Here's how the part is built. I have some questions about the finished solid (model axes, mm). Face numbers are marked on the shaded views. A direction names the side the tool comes from. Round coordinates to 2 decimals unless told otherwise and drop trailing zeros. Order: outer loops, then holes, each group sorted by start corner. A loop starts at its lowest first (then second) coordinate and runs counter-clockwise, first axis right, second up. Notation, with made-up numbers: (-22, 1) - (-2, 1) arc R17 cw to (-2, 12) - close; hole circle Ø2 at (56, 82.25). An arc over 180 degrees is marked (long way). One line per item, written item: value.
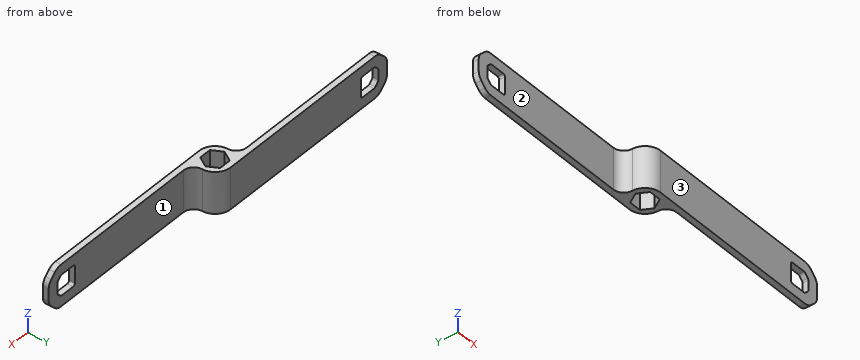
from build123d import *

# Parameters (mm, degrees)
SKETCH2_R           = 7.5
BOSS_EXTRUDE1_DEPTH = 20
SKETCH3_W           = 20
SKETCH3_H           = 2.7375
BOSS_EXTRUDE2_DEPTH = 90
FILLET1_R           = 5
CHAMFER1_SIZE       = 5
FILLET2_R           = 5
CUT_EXTRUDE1_DEPTH  = 45
FILLET3_R           = 1
SKETCH5_W           = 20
SKETCH5_H           = 2.7375
BOSS_EXTRUDE3_DEPTH = 90
CHAMFER2_SIZE       = 5
FILLET4_R           = 5
FILLET5_R           = 5
CUT_EXTRUDE2_DEPTH  = 90
FILLET6_R           = 1


with BuildPart() as part:
    # Sketch2 → Boss-Extrude1 (new body)
    with BuildSketch(Plane.XY):
        Circle(SKETCH2_R)
        Polygon((5.499261314, 0), (2.749630657, 4.7625), (-2.749630657, 4.7625), (-5.499261314, 0), (-2.749630657, -4.7625), (2.749630657, -4.7625), align=None, mode=Mode.SUBTRACT)
    extrude(amount=BOSS_EXTRUDE1_DEPTH)

    # Sketch3 → Boss-Extrude2 (add)
    with BuildSketch(Plane.ZY):
        with Locations((10, 6.13125)):
            Rectangle(SKETCH3_W, SKETCH3_H)
    extrude(amount=BOSS_EXTRUDE2_DEPTH)

    # Fillet1
    fillet1_edges = [part.edges().sort_by_distance(p)[0] for p in [
        (-5.793841019, 4.7625, 10),
    ]]
    fillet(fillet1_edges, radius=FILLET1_R)

    # Chamfer1
    chamfer1_edges = [part.edges().sort_by_distance(p)[0] for p in [
        (-90, 6.13125, 0),
        (-90, 6.13125, 20),
    ]]
    chamfer(chamfer1_edges, length=CHAMFER1_SIZE)

    # Fillet2
    fillet2_edges = [part.edges().sort_by_distance(p)[0] for p in [
        (-90, 6.13125, 15),
        (-90, 6.13125, 5),
        (-85, 6.13125, 0),
        (-85, 6.13125, 20),
    ]]
    fillet(fillet2_edges, radius=FILLET2_R)

    # Sketch4 → Cut-Extrude1 (cut)
    with BuildSketch(Plane(origin=(0, 7.5, 0), x_dir=(1, 0, 0), z_dir=(0, 1, 0))):
        Polygon((-74.928932188, -15), (-74.928932188, -5), (-82.928932188, -5), (-85, -7.071067812), (-85, -12.928932188), (-82.928932188, -15), align=None)
    extrude(amount=-CUT_EXTRUDE1_DEPTH, mode=Mode.SUBTRACT)

    # Fillet3
    fillet3_edges = [part.edges().sort_by_distance(p)[0] for p in [
        (-74.928932188, 6.13125, 15),
        (-82.928932188, 6.13125, 15),
        (-85, 6.13125, 12.928932188),
        (-85, 6.13125, 7.071067812),
        (-82.928932188, 6.13125, 5),
        (-74.928932188, 6.13125, 5),
    ]]
    fillet(fillet3_edges, radius=FILLET3_R)

    # Sketch5 → Boss-Extrude3 (add)
    with BuildSketch(Plane.ZY):
        with Locations((10, -6.13125)):
            Rectangle(SKETCH5_W, SKETCH5_H)
    extrude(amount=-BOSS_EXTRUDE3_DEPTH)

    # Chamfer2
    chamfer2_edges = [part.edges().sort_by_distance(p)[0] for p in [
        (90, -6.13125, 20),
        (90, -6.13125, 0),
    ]]
    chamfer(chamfer2_edges, length=CHAMFER2_SIZE)

    # Fillet4
    fillet4_edges = [part.edges().sort_by_distance(p)[0] for p in [
        (85, -6.13125, 20),
        (90, -6.13125, 5),
        (90, -6.13125, 15),
        (85, -6.13125, 0),
    ]]
    fillet(fillet4_edges, radius=FILLET4_R)

    # Fillet5
    fillet5_edges = [part.edges().sort_by_distance(p)[0] for p in [
        (5.793841019, -4.7625, 10),
    ]]
    fillet(fillet5_edges, radius=FILLET5_R)

    # Sketch7 → Cut-Extrude2 (cut)
    with BuildSketch(Plane.XZ.offset(7.5)):
        Polygon((74.928932188, 5), (74.928932188, 15), (82.928932188, 15), (85, 12.928932188), (85, 7.071067812), (82.928932188, 5), align=None)
    extrude(amount=-CUT_EXTRUDE2_DEPTH, mode=Mode.SUBTRACT)

    # Fillet6
    fillet6_edges = [part.edges().sort_by_distance(p)[0] for p in [
        (82.928932188, -6.13125, 5),
        (74.928932188, -6.13125, 5),
        (74.928932188, -6.13125, 15),
        (82.928932188, -6.13125, 15),
        (85, -6.13125, 12.928932188),
        (85, -6.13125, 7.071067812),
    ]]
    fillet(fillet6_edges, radius=FILLET6_R)


solid = part.part
Q1. If I drill on line 1 along Y through (x, z) = (-26.5, 10.5); line 2 along Y through (x, z) = (45.5, 3); line 3 along X through (y, z) = (2, 9.25), over which ranges is the centre line in solid material (lowest first)?
Results list:
line 1: 4.76 to 7.5
line 2: -7.5 to -4.76
line 3: -8.03 to -4.34, 4.34 to 7.23
Q2. If we section it at A-A, the plane x = -54: Please give me the cut outline in (y, z).
Results list:
outline: (4.76, 0) - (7.5, 0) - (7.5, 20) - (4.76, 20) - close
Q3. Which directions (+Z, -Z, +X, -X, +Y, -Y) give clear straight access to the entire face, cutting with the end or side of a thin tool? Please do the marked faces 1, 2 and 3.
Results list:
face 1: +Z, -Z, +X, +Y
face 2: +Z, -Z, -X, -Y
face 3: +Z, -Z, +X, -X, -Y
Q4. If we section it at B-B, the plane x = 11: Please give me the cut outline in (y, z), then the cut area to 3 significant figures.
Results list:
outline: (-7.5, 0) - (-4.53, 0) - (-4.53, 20) - (-7.5, 20) - close
area: 59.3 mm²
Q5. Will these pins go through, and if not, where does the flat tip stop? pin 1 (6 mm diameter, centred on x = 67, z = 9, fed in from +Y); pin 2 (6 mm diameter, centred on x = -47.5, z = 9, fed in from -Y); pin 3 (1.4 mm diameter, centred on y = -6, z = 10, fed in from -X).
Results list:
pin 1: y = -4.76
pin 2: y = 4.76
pin 3: x = -5.31
